Input: dimensioned drawing with shaded views. Units: mm. Origin: part minimum x, y, z. Round coordinates to 2 decimals unless told otherwise and drop trailing zeros. Order: outer loops, then holes, each group sorted by start corner. A loop starts at its lowest first (then second) coordinate and runs counter-clockwise, first axis right, second up. Notation, with made-up numbers: M 47.5,-1 L 51.5,-1 A23 cw 51.5,11 Z; hole C -1.75,29 d2. An arc over 180 degrees is marked long. Answer as CSV lines item,"result". Start each with the question number.
Item 1: First-contact query: P1, Ø2.5, axis at x = 18.5, y = 22.16, coming from the -Z side; P2, Ø10, axis at x = 16, y = 10.5, coming from the -Z side. Flat tips, straight axial feed; report the tip coordinate or a pass-through.
Item 2: Section query C-C on z = 7.25. State how many separate pieces and enclosed holes the cut face has, plus the area to 3 significant figures.
Item 3: Section query A-A on y = 13.5. Return the cut outline in (x, z).
Item 4: Pull-direction query (X, two-part tool) for the marked faces 1, 2, 3 and 4; classes: +X half, -X half, draft (parallel to the pull), parting line (faces both ways), or undercut.
Item 5: Section query D-D on x = 2.5. Return the cut outline in (y, z).
Item 6: Line query: line 1 (X direction, y = 9.5, z = 7.5) (1 decimal); line 2 (Y direction, x = 22.75, z = 4.5); line 3 (X direction, y = 23.25, z = 4). Output: solid intervals per line, ascending. Write a range as [from, to].
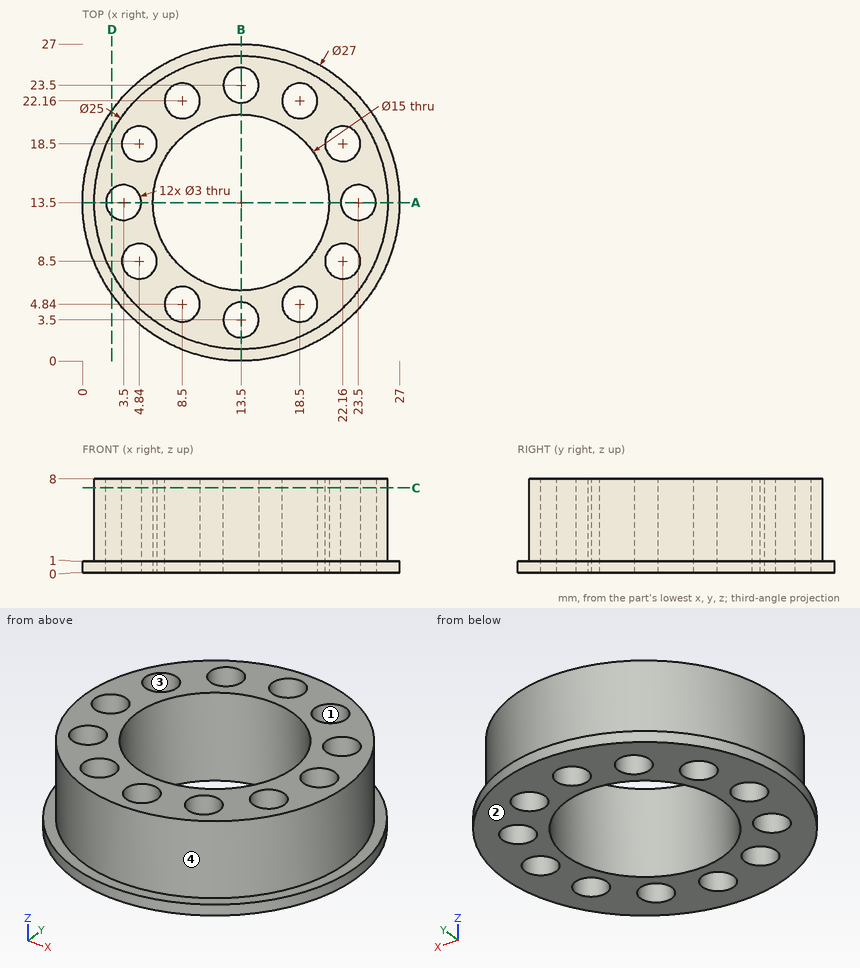
Results:
1,P1,"through"
1,P2,"z = 0"
2,separate pieces,"1"
2,enclosed holes,"13"
2,area,"229 mm^2"
3,outline,"M 0,0 L 2,0 L 2,8 L 1,8 L 1,1 L 0,1 Z; M 5,0 L 6,0 L 6,8 L 5,8 Z; M 21,0 L 22,0 L 22,8 L 21,8 Z; M 25,0 L 27,0 L 27,1 L 26,1 L 26,8 L 25,8 Z"
4,face 1,"undercut"
4,face 2,"draft"
4,face 3,"undercut"
4,face 4,"parting line"
5,outline,"M 5.67,0 L 12.38,0 L 12.38,8 L 7.56,8 L 7.56,1 L 5.67,1 Z; M 14.62,0 L 21.33,0 L 21.33,1 L 19.44,1 L 19.44,8 L 14.62,8 Z"
6,line 1,"[1.7, 3.7], [6, 7.2], [19.8, 21], [23.3, 25.3]"
6,line 2,"[5.09, 7.12], [9.88, 12.2], [14.8, 17.12], [19.88, 21.91]"
6,line 3,"[5.68, 7.47], [9.53, 12.02], [14.98, 17.47], [19.53, 21.32]"
